Study the drawing (mm; zero at the part's minimum x, y, z) and answer. Round coordinates to 2 decimals unless told otherwise and drop trailing zeros. Write each loop counter-clockwise with the first axis right and the second up, starting at its lowest first coordinate (ties: lowest second). Pieces come first, ordered by that corner, then holes.
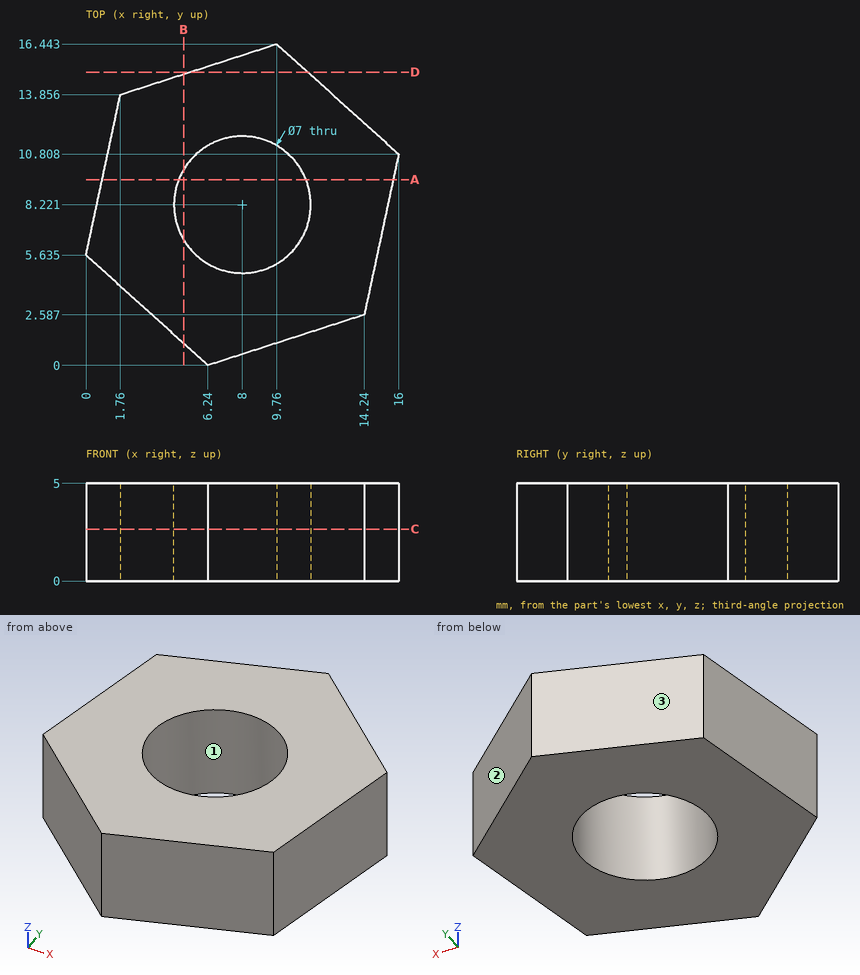
1. Section C-C on z = 2.65 is taken. Determine the outline of the cut face in (x, y) (1 decimal).
Geometry says:
outline: (0, 5.6) - (6.2, 0) - (14.2, 2.6) - (16, 10.8) - (9.8, 16.4) - (1.8, 13.9) - close; hole circle Ø7 at (8, 8.2)
2. Section A-A on y = 9.5 is taken. Determine the outline of the cut face in (x, z).
Geometry says:
outline: (0.83, 0) - (4.74, 0) - (4.74, 5) - (0.83, 5) - close; (11.26, 0) - (15.72, 0) - (15.72, 5) - (11.26, 5) - close
3. Section B-B on x = 5 is taken. Determine the outline of the cut face in (y, z) (1 decimal).
Geometry says:
outline: (1.1, 0) - (6.4, 0) - (6.4, 5) - (1.1, 5) - close; (10, 0) - (14.9, 0) - (14.9, 5) - (10, 5) - close
4. For a pull along X with two mould halves and no side action, classify the marked faces 1, 2 and 3 as released by +X, released by -X, zero draft, split by the parting line, or undercut.
Geometry says:
face 1: undercut
face 2: released by +X
face 3: released by -X
5. Section D-D on y = 15 is taken. Determine the outline of the cut face in (x, z), plus the area to 3 significant figures.
Geometry says:
outline: (5.3, 0) - (11.36, 0) - (11.36, 5) - (5.3, 5) - close
area: 30.3 mm2
6. Given pin 1 (3 mm diameter, centred on y = 12, z = 4.5, fed in from -X); pin 2 (1 mm diameter, centred on y = 7, z = 1, fed in from +X), each flat-ended and moving along its own axis, determine where each tip first touches the part or whether it passes through.
Geometry says:
pin 1: stops at x = 1.04
pin 2: stops at x = 15.29
7. Straight lines are drawn through the part: line 1 along Y through (x, z) = (8, 1.8) (1 decimal); line 2 along Y through (x, z) = (10.5, 0.85) (1 decimal); line 3 along X through (y, z) = (7.75, 2.85) (1 decimal). For each, find the intervals that lie inside material, in ascending order.
Geometry says:
line 1: y = 0.6 to 4.7, 11.7 to 15.9
line 2: y = 1.4 to 5.8, 10.7 to 15.8
line 3: x = 0.5 to 4.5, 11.5 to 15.3
